```python
from build123d import *

# Parameters (mm, degrees)
SKETCH2_R           = 30
BOSS_EXTRUDE1_DEPTH = 10
SKETCH3_R           = 25
SKETCH3_R_2         = 5
CUT_EXTRUDE1_DEPTH  = 3
SKETCH4_R           = 5
CUT_EXTRUDE2_DEPTH  = 44
CHAMFER1_SIZE       = 0.1


# Read off the part's stored shape, not the designer's step: Cut-Revolve1
with BuildPart() as part:
    # Sketch2 → Boss-Extrude1 (new body)
    with BuildSketch(Plane.XY):
        Circle(SKETCH2_R)
    extrude(amount=BOSS_EXTRUDE1_DEPTH)

    # Sketch3 → Cut-Extrude1 (cut)
    with BuildSketch(Plane.XY.offset(10)):
        Circle(SKETCH3_R)
        Circle(SKETCH3_R_2, mode=Mode.SUBTRACT)
    cut_extrude1 = extrude(amount=-CUT_EXTRUDE1_DEPTH, mode=Mode.SUBTRACT)

    # Mirror2: Cut-Extrude1 across plane
    add(cut_extrude1.mirror(Plane.XY.offset(5)), mode=Mode.SUBTRACT)

    # Sketch4 → Cut-Extrude2 (cut, through all)
    with BuildSketch(Plane.XY.offset(7)):
        with Locations((0, 17)):
            Circle(SKETCH4_R)
        with Locations((12.02081528, 12.02081528)):
            Circle(SKETCH4_R)
        with Locations((17, 0)):
            Circle(SKETCH4_R)
        with Locations((12.02081528, -12.02081528)):
            Circle(SKETCH4_R)
        with Locations((0, -17)):
            Circle(SKETCH4_R)
        with Locations((-12.02081528, -12.02081528)):
            Circle(SKETCH4_R)
        with Locations((-17, 0)):
            Circle(SKETCH4_R)
        with Locations((-12.02081528, 12.02081528)):
            Circle(SKETCH4_R)
    extrude(amount=-CUT_EXTRUDE2_DEPTH, mode=Mode.SUBTRACT)

    # Chamfer1
    chamfer1_edges = [part.edges().sort_by_distance(p)[0] for p in [
        (-25, 0, 0),
        (-17.02081528, 12.02081528, 7),
        (-22, 0, 7),
        (-17.02081528, -12.02081528, 7),
        (-5, -17, 7),
        (7.02081528, -12.02081528, 7),
        (12, 0, 7),
        (7.02081528, 12.02081528, 7),
        (-5, 17, 7),
        (-30, 0, 10),
        (-25, 0, 7),
        (-25, 0, 10),
        (-5, 0, 10),
    ]]
    chamfer(chamfer1_edges, length=CHAMFER1_SIZE)

    # Cut-Revolve1 outline → Cut-Revolve1 (revolve, cut)
    with BuildSketch(Plane.XZ):
        Polygon((2, 0), (2, 6), (1.5, 6), (1.5, 8.5), (3, 10), (0, 10), (0, 0), align=None)
    revolve(axis=Axis((0, 0, 0), (0, 0, 1)), mode=Mode.SUBTRACT)


solid = part.part
```
Source: CAD feature listing. Evaluate the final solid. Frame: model axes, mm. A direction names the side the tool comes from. Give positions to 0.01 mm unless a question says otherwise; leave off trailing zeros. Loops run counter-clockwise (first coordinate to the right, second up) from the corner with the lowest first, then second, coordinate; pieces in that order, holes last. Notation, with made-up numbers: (18.25, 24.25) -> (22.25, 24.25) arc R12 ccw to (22.25, 35.25) -> close; hole circle Ø3 at (38, 65). An arc over 180 degrees is marked (long way). Use a Markdown table: item, result. Add a question column.
(1) Section query A-A (z = 2). Output: boundary loops of the cut face in (x, y).
(2) Pull-direction query (X, two-part tool) for faces 4 (the face through (-29.97, 1.32, 4.88)), 5 (the face through (2.2, 0.1, 0)), 6 (the face through (-0.3, -5.2, 7)); classes: +X half, -X half, draft (parallel to the pull), parting line (faces both ways), or undercut.
(3) Access query for faces 1 (the face through (0, -2, 3)), 2 (the face through (23.846, 7.509, 8.52)), 3 (the face through (-0.1, -3.2, 10)). Directions: +Z, -Z, +X, -X, +Y, -Y. A direction counts if a zero-diameter tool reaches every point of the face in a straight line with its end or side. Return the directions, or none.
(4) Ray query, line 1 (Y direction, x = 0, z = 1.95); line 2 (Y direction, x = 9.5, z = 4.25); line 3 (X direction, y = 16.5, z = 4). Return the intervals inside material, ascending.
(5) Section query B-B (x = 0). Count the separate pieces of the cut face and the enclosed holes in it, then the cut area to 3 significant figures.
(6) First-contact query: pin 1 Ø1.5 at (x, z) = (23.5, 1.5) entering from -Y; pin 2 Ø13 at (x, y) = (-12.02, 12.02) entering from -Z; pin 3 Ø2 at (y, z) = (-5.5, 6) entering from +X; pin 4 Ø6 at (x, y) = (17, 0) entering from +Z. Flat tips, straight axial feed; report the tip coordinate or a pass-through.
Checked values:
| question | item | result |
|---|---|---|
| 1 | outline | circle Ø60 at (0, 0); circle Ø10 at (0, 0); hole circle Ø50 at (0, 0); hole circle Ø4 at (0, 0) |
| 2 | face 4 | parting line |
| 2 | face 5 | draft |
| 2 | face 6 | undercut |
| 3 | face 1 | -Z |
| 3 | face 2 | +Z |
| 3 | face 3 | +Z, +X, -X, +Y, -Y |
| 4 | line 1 | -30 to -25, -5 to -2, 2 to 5, 25 to 30 |
| 4 | line 2 | -28.46 to -16.34, -7.7 to 7.7, 16.34 to 28.46 |
| 4 | line 3 | -25.05 to -14.24, -9.8 to -4.97, 4.97 to 9.8, 14.24 to 25.05 |
| 5 | separate pieces | 4 |
| 5 | enclosed holes | 0 |
| 5 | area | 242 mm^2 |
| 6 | pin 1 | y = -19.56 |
| 6 | pin 2 | z = 3 |
| 6 | pin 3 | x = 29.66 |
| 6 | pin 4 | through |
